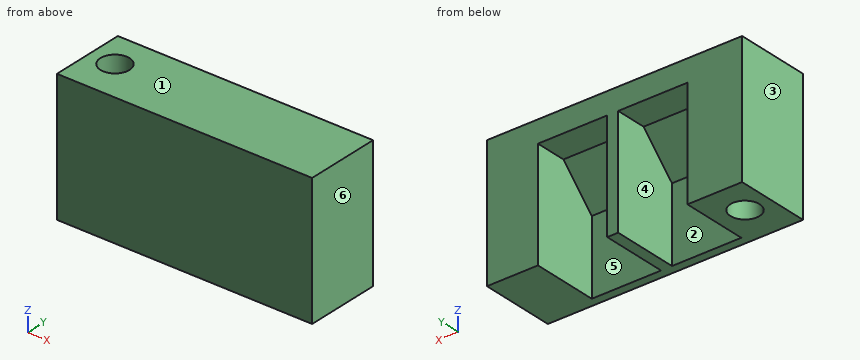
from build123d import *

# Parameters (mm, degrees)
CYLINDER003_R     = 2
CYLINDER003_DEPTH = 20
BOX007_W          = 36
BOX007_H          = 10
BOX007_DEPTH      = 10
BOX007_ROLL_ANGLE = 45
BOX006_W          = 9.5
BOX006_H          = 10
BOX006_DEPTH      = 15
BOX004_W          = 9.5
BOX004_H          = 10
BOX004_DEPTH      = 15
BOX001_W          = 35
BOX001_H          = 10.3
BOX001_DEPTH      = 18


with BuildPart() as zylinder003:
    # Cylinder003 → Cylinder003 (new body)
    with BuildSketch(Plane(origin=(6, -4.5, -12), x_dir=(1, 0, 0), z_dir=(0, 0, 1))):
        Circle(CYLINDER003_R)
    extrude(amount=CYLINDER003_DEPTH)


with BuildPart() as obj1:
    # Box007 → Box007 (new body)
    with BuildSketch(Plane.XY):
        with Locations((18, 5)):
            Rectangle(BOX007_W, BOX007_H)
    extrude(amount=BOX007_DEPTH)


with BuildPart() as obj1_1:
    # Box007 roll: moved
    add(obj1.part.rotate(Axis((0, 0, 0), (1, 0, 0)), BOX007_ROLL_ANGLE))


with BuildPart() as obj1_2:
    # Box007 placement: moved
    add(obj1_1.part.moved(Location((0, -10, -2))))


with BuildPart() as obj2:
    # Box006 → Box006 (new body)
    with BuildSketch(Plane(origin=(21, -8.8, -11), x_dir=(1, 0, 0), z_dir=(0, 0, 1))):
        with Locations((4.75, 5)):
            Rectangle(BOX006_W, BOX006_H)
    extrude(amount=BOX006_DEPTH)


with BuildPart() as cut001:
    # Box004 → Box004 (new body)
    with BuildSketch(Plane(origin=(10, -8.8, -11), x_dir=(1, 0, 0), z_dir=(0, 0, 1))):
        with Locations((4.75, 5)):
            Rectangle(BOX004_W, BOX004_H)
    extrude(amount=BOX004_DEPTH)

    # Fusion007: union obj2
    add(obj2.part)

    # Cut001: cut obj1
    add(obj1_2.part, mode=Mode.SUBTRACT)


with BuildPart() as cut003:
    # Box001 → Box001 (new body)
    with BuildSketch(Plane(origin=(2.5, -10, -11), x_dir=(1, 0, 0), z_dir=(0, 0, 1))):
        with Locations((17.5, 5.15)):
            Rectangle(BOX001_W, BOX001_H)
    extrude(amount=BOX001_DEPTH)

    # Cut002: cut Cut001
    add(cut001.part, mode=Mode.SUBTRACT)

    # Cut003: cut Zylinder003
    add(zylinder003.part, mode=Mode.SUBTRACT)


solid = cut003.part
Input: part model. Units: mm. Frame: model coordinates. Face numbers are marked on the shaded views. A direction names the side the tool comes from. Coordinates: 2 decimals unless noted, no trailing zeros. Loops run counter-clockwise (first coordinate to the right, second up) from the corner with the lowest first, then second, coordinate; pieces in that order, holes last.
Q1. Contact query for flat-ended pins moving along their axis: pin 1 (2 mm diameter, centred on x = 26, z = 1.5, fed in from +Y); pin 2 (3.5 mm diameter, centred on x = 28, y = -3, fed in from -Z); pin 3 (1.3 mm diameter, centred on x = 15, y = -1.5, fed in from -Z). Output: stop coordinate, or through.
Q2. Material intervals for line 1 (X direction, y = -7.5, z = -7.5); line 2 (Y direction, x = 6, z = -4.75); line 3 (X direction, y = -6, z = -6.5), sorted ascending.
Q3. Cut plane A-A (y = -4.5). Output: boundary loops of the cut face in (x, z).
Q4. Set-up query: the marked faces 1 and 2. Return all of +Z, -Z, +X, -X, +Y, -Y with unobstructed straight access to the full face (end or side cutting, diameter ignored); none if empty.
Q5. Cut plane D-D (x = 30). Output: boundary loops of the cut face in (y, z), then the cut area to 3 significant figures.
Q6. Cut plane B-B (z = 0). Output: boundary loops of the cut face in (x, y).
Q7. Draft query along X for the marked faces 3, 4, 5 and 6. Return one class per face: +X half, -X half, draft (parallel to the pull), parting line (faces both ways), or undercut.
Q8. Cut plane C-C (x = 6). Output: boundary loops of the cut face in (y, z), then the cut area to 3 significant figures.
Working result:
1. pin 1: stops at y = -5.5
1. pin 2: stops at z = 3.25
1. pin 3: stops at z = 4
2. line 1: x = 2.5 to 10, 19.5 to 21, 30.5 to 37.5
2. line 2: y = -10 to -6.5, -2.5 to 0.3
2. line 3: x = 2.5 to 4.68, 7.32 to 10, 19.5 to 21, 30.5 to 37.5
3. outline: (2.5, -11) - (4, -11) - (4, 7) - (2.5, 7) - close; (8, -11) - (10, -11) - (10, 3.5) - (19.5, 3.5) - (19.5, -11) - (21, -11) - (21, 3.5) - (30.5, 3.5) - (30.5, -11) - (37.5, -11) - (37.5, 7) - (8, 7) - close
4. face 1: +Z, +X, -X, +Y, -Y
4. face 2: -Z, +Y
5. outline: (-10, -11) - (-8.8, -11) - (-8.8, -0.8) - (-4, 4) - (0.3, 4) - (0.3, 7) - (-10, 7) - close
5. area: 60.4 mm2
6. outline: (2.5, -10) - (37.5, -10) - (37.5, 0.3) - (30.5, 0.3) - (30.5, -8) - (21, -8) - (21, 0.3) - (19.5, 0.3) - (19.5, -8) - (10, -8) - (10, 0.3) - (2.5, 0.3) - close; hole circle Ø4 at (6, -4.5)
7. face 3: -X half
7. face 4: undercut
7. face 5: undercut
7. face 6: +X half
8. outline: (-10, -11) - (-6.5, -11) - (-6.5, 7) - (-10, 7) - close; (-2.5, -11) - (0.3, -11) - (0.3, 7) - (-2.5, 7) - close
8. area: 113 mm2
